from build123d import *

# Parameters (mm, degrees)
BASEFLANGE_W                   = 50
BASEFLANGE_H                   = 640
BASE_FLANGE1_DEPTH             = 2
EDGE_FLANGE1_STRIP_W           = 10
EDGE_FLANGE1_STRIP_H           = 2
EDGE_FLANGE1_STRIP_CUT_DEPTH   = 50
EDGE_FLANGE1_STRIP_2_W         = 10
EDGE_FLANGE1_STRIP_2_H         = 2
EDGE_FLANGE1_STRIP_CUT_2_DEPTH = 50
EDGE_FLANGE1_DEPTH             = 50
EDGE_FLANGE1_BEND_DEPTH        = 50
SKETCH8_R                      = 4.6
EXTRUDE1_DEPTH                 = 642.190299365


# Sheet-metal steps are written as plain solids
with BuildPart() as part:
    # BaseFlange → Base-Flange1 (new body)
    with BuildSketch(Plane(origin=(0, 0, 0), x_dir=(1, 0, 0), z_dir=(0, 1, 0))):
        Rectangle(BASEFLANGE_W, BASEFLANGE_H)
    extrude(amount=BASE_FLANGE1_DEPTH)

    # Edge-Flange1 strip (across the edge) → Edge-Flange1 strip cut (cut)
    with BuildSketch(Plane(origin=(-25, 2, 320), x_dir=(0, 0, -1), z_dir=(1, 0, 0))):
        with Locations((-2, -1)):
            Rectangle(EDGE_FLANGE1_STRIP_W, EDGE_FLANGE1_STRIP_H)
    extrude(amount=EDGE_FLANGE1_STRIP_CUT_DEPTH, mode=Mode.SUBTRACT)

    # Edge-Flange1 strip 2 (across the edge) → Edge-Flange1 strip cut 2 (cut)
    with BuildSketch(Plane(origin=(25, 2, -320), x_dir=(0, 0, 1), z_dir=(-1, 0, 0))):
        with Locations((-2, -1)):
            Rectangle(EDGE_FLANGE1_STRIP_2_W, EDGE_FLANGE1_STRIP_2_H)
    extrude(amount=EDGE_FLANGE1_STRIP_CUT_2_DEPTH, mode=Mode.SUBTRACT)

    # Edge-Flange1 section (across the edge) → Edge-Flange1 (add)
    with BuildSketch(Plane(origin=(-25, 2, 320), x_dir=(0, 0, -1), z_dir=(1, 0, 0))):
        with BuildLine():
            Line((0, 1), (0, 28))
            Line((0, 28), (2, 28))
            Line((2, 28), (2, 1))
            ThreePointArc((2, 1), (2.292893219, 0.292893219), (3, 0))
            Line((3, 0), (3, -2))
            ThreePointArc((3, -2), (0.878679656, -1.121320344), (0, 1))
        make_face()
    extrude(amount=EDGE_FLANGE1_DEPTH)

    # Edge-Flange1 section 2 (across the edge) → Edge-Flange1 bend (add)
    with BuildSketch(Plane(origin=(25, 2, -320), x_dir=(0, 0, 1), z_dir=(-1, 0, 0))):
        with BuildLine():
            Line((0, 1), (0, 28))
            Line((0, 28), (2, 28))
            Line((2, 28), (2, 1))
            ThreePointArc((2, 1), (2.292893219, 0.292893219), (3, 0))
            Line((3, 0), (3, -2))
            ThreePointArc((3, -2), (0.878679656, -1.121320344), (0, 1))
        make_face()
    extrude(amount=EDGE_FLANGE1_BEND_DEPTH)

    # Sketch8 → Extrude1 (cut, through all)
    with BuildSketch(Plane.XY.offset(320)):
        with Locations((0, 15)):
            Circle(SKETCH8_R)
    extrude(amount=-EXTRUDE1_DEPTH, mode=Mode.SUBTRACT)


solid = part.part
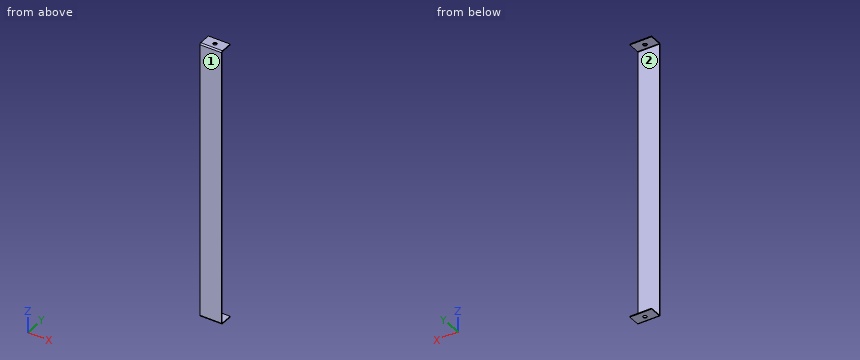
CAD build for the part. Positions are in the model's coordinates, mm. Face numbers are marked on the shaded views. A direction names the side the tool comes from. Round coordinates to 2 decimals unless told otherwise and drop trailing zeros. Loops run counter-clockwise (first coordinate to the right, second up) from the corner with the lowest first, then second, coordinate; pieces in that order, holes last.
(1) Which spindle directions (+Z, -Z, +X, -X, +Y, -Y) get a long thin tool onto all of the face, cutting with end or side? Do the marked faces 1 and 2. Say none if no direction does.
(2) Drop a flat-ended pin along its axis: pin 1 (6 mm diameter, centred on x = 17.5, z = 229.5, fed in from +Y). Give the stop position or say it passes through.
(3) Cut at B-B (x = -17). Give the cut face in (y, z).
(4) Cut at A-A (y = 15). Give the cut face in (x, z), plus the area to 3 significant figures.
(5) Wall check: line 1 along Z through (x, y) = (14, 19.5); line 2 along Y through (x, z) = (3.5, 79); line 3 along Y through (x, z) = (0, 319). Give the ranges that are in metal, low to high.
(6) Cut at C-C (z = 263). Give the cut face in (x, y), plus the area to 3 significant figures.
Findings below:
1. face 1: +Z, -Z, +X, -X, -Y
1. face 2: +X, -X, +Y
2. pin 1: stops at y = 2
3. outline: (0, -317) arc R3 ccw to (3, -320) - (30, -320) - (30, -318) - (3, -318) arc R1 cw to (2, -317) - (2, 317) arc R1 cw to (3, 318) - (30, 318) - (30, 320) - (3, 320) arc R3 ccw to (0, 317) - close
4. outline: (-25, -320) - (-4.6, -320) - (-4.6, -318) - (-25, -318) - close; (-25, 318) - (-4.6, 318) - (-4.6, 320) - (-25, 320) - close; (4.6, -320) - (25, -320) - (25, -318) - (4.6, -318) - close; (4.6, 318) - (25, 318) - (25, 320) - (4.6, 320) - close
4. area: 163 mm2
5. line 1: z = -320 to -318, 318 to 320
5. line 2: y = 0 to 2
5. line 3: y = 0.76 to 10.4, 19.6 to 30
6. outline: (-25, 0) - (25, 0) - (25, 2) - (-25, 2) - close
6. area: 100 mm2
